Can you work these out from the model? Positions are in its coordinate system, mm. Face numbers are marked on the shaded views. A direction names the side the tool comes from. Round coordinates to 2 decimals unless told otherwise and drop trailing zeros. Order: outer loops, then holes, each group sorted by start corner. A loop starts at its lowest first (then second) coordinate and runs counter-clockwise, first axis right, second up. Notation, with made-up numbers: (-28, -28.75) -> (3, -28.75) arc R24 cw to (3, -16.75) -> close; hole circle Ø5 at (-1, 78). An arc over 180 degrees is marked (long way). Use a Markdown table: item, result. Add a question column.
Q1. For the marked faces 1, 2, 3, 4 and 5, which set-ups out of +Z, -Z, +X, -X, +Y, -Y let a thin tool reach every point of the face, with its end or its side?
Q2. I'm going to push flat-ended pins straight in: pin 1 Ø15 at (x, y) = (13, 13.5) entering from +Z; pin 2 Ø1.8 at (x, y) = (-50, 14) entering from +Z; pin 3 Ø2 at (y, z) = (9.5, -22) entering from +X. Where does each tip first touch, or does it pass through?
Q3. If we section it at C-C on x = -34.5: List the corners of the cut face in (y, z) for me, plus the area to 3 significant figures.
Q4. If we section it at D-D on z = -5: List the corners of the cut face in (x, y) for me.
Q5. We'd pull the mould along X, two halves only. Please class the marked faces 6, 7 and 8: +X half, -X half, draft (parallel to the pull), parting line (faces both ways), or undercut.
Q6. If we section it at A-A on z = 8.5: List the corners of the cut face in (x, y) for me.
Q7. I need wall thicknesses on line 1 along X through (y, z) = (12, 45.5); line 2 along X through (y, z) = (2.5, 21.5); line 3 along Z through (x, y) = (-25, 3). Which ranges of each line are inside material? Lowest first, please. Write a range as [from, to].
Q8. If we section it at B-B on y = 11: List the corners of the cut face in (x, z) for me, plus the area to 3 significant figures.
```python
from build123d import *

# Parameters (mm, degrees)
AUFSATZ_LINEAR_AUSTRAGEN1_DEPTH = 30
SKIZZE5_W                       = 8.1
SKIZZE5_H                       = 30
AUFSATZ_LINEAR_AUSTRAGEN2_DEPTH = 3
FASE2_SIZE                      = 0.5
VERRUNDUNG1_R                   = 5
VERRUNDUNG2_R                   = 10
SCHNITT_LINEAR_AUSTRAGEN1_DEPTH = 135.433068848
VERRUNDUNG3_R                   = 2
SCHNITT_LINEAR_AUSTRAGEN2_DEPTH = 97.953597148
SCHNITT_LINEAR_AUSTRAGEN3_DEPTH = 103.097992145


with BuildPart() as part:
    # Skizze1 → Aufsatz-Linear austragen1 (new body)
    with BuildSketch(Plane(origin=(0, 0, 0), x_dir=(1, 0, 0), z_dir=(0, 1, 0))):
        Polygon((-56.5, 0), (-56.5, -26), (-46.5, -26), (-46.5, 8), (60, 8), (60, -60), (70, -60), (70, 0), (70, 20), (-56.5, 20), align=None)
    extrude(amount=AUFSATZ_LINEAR_AUSTRAGEN1_DEPTH)

    # Skizze5 → Aufsatz-Linear austragen2 (add)
    with BuildSketch(Plane(origin=(0, 0, -20), x_dir=(-1, 0, 0), z_dir=(0, 0, -1))):
        with Locations((0, 15)):
            Rectangle(SKIZZE5_W, SKIZZE5_H)
    extrude(amount=AUFSATZ_LINEAR_AUSTRAGEN2_DEPTH)

    # Fase2
    fase2_edges = [part.edges().sort_by_distance(p)[0] for p in [
        (-4.05, 15, -23),
        (0, 0, -23),
        (4.05, 15, -23),
        (0, 30, -23),
    ]]
    chamfer(fase2_edges, length=FASE2_SIZE)

    # Verrundung1
    verrundung1_edges = [part.edges().sort_by_distance(p)[0] for p in [
        (70, 15, -20),
        (-56.5, 15, -20),
    ]]
    fillet(verrundung1_edges, radius=VERRUNDUNG1_R)

    # Verrundung2
    verrundung2_edges = [part.edges().sort_by_distance(p)[0] for p in [
        (60, 15, -8),
        (-46.5, 15, -8),
    ]]
    fillet(verrundung2_edges, radius=VERRUNDUNG2_R)

    # Skizze8 → Schnitt-Linear austragen1 (cut, through all)
    with BuildSketch(Plane.ZY.offset(-60)):
        Polygon((17, 26.65), (15.35, 25), (17, 23.35), (18.65, 25), align=None)
        Polygon((48.35, 25), (50, 26.65), (51.65, 25), (50, 23.35), align=None)
    extrude(amount=-SCHNITT_LINEAR_AUSTRAGEN1_DEPTH, mode=Mode.SUBTRACT)

    # Verrundung3
    verrundung3_edges = [part.edges().sort_by_distance(p)[0] for p in [
        (70, 15, 60),
        (60, 15, 60),
        (-46.5, 15, 26),
        (-56.5, 15, 26),
    ]]
    fillet(verrundung3_edges, radius=VERRUNDUNG3_R)

    # Skizze9 → Schnitt-Linear austragen2 (cut, through all)
    with BuildSketch(Plane(origin=(0, 0, 0), x_dir=(0, 0, -1), z_dir=(1, 0, 0))):
        Polygon((-16, 27.192031022), (-13.807968978, 25), (-16, 22.807968978), (-18.192031022, 25), align=None)
        Polygon((-16, 7.192031022), (-13.807968978, 5), (-16, 2.807968978), (-18.192031022, 5), align=None)
    extrude(amount=-SCHNITT_LINEAR_AUSTRAGEN2_DEPTH, mode=Mode.SUBTRACT)

    # Skizze10 → Schnitt-Linear austragen3 (cut, through all)
    with BuildSketch(Plane.XY.offset(-8)):
        Polygon((0, 17.55), (2.55, 15), (0, 12.45), (-2.55, 15), align=None)
    extrude(amount=-SCHNITT_LINEAR_AUSTRAGEN3_DEPTH, mode=Mode.SUBTRACT)


solid = part.part
```
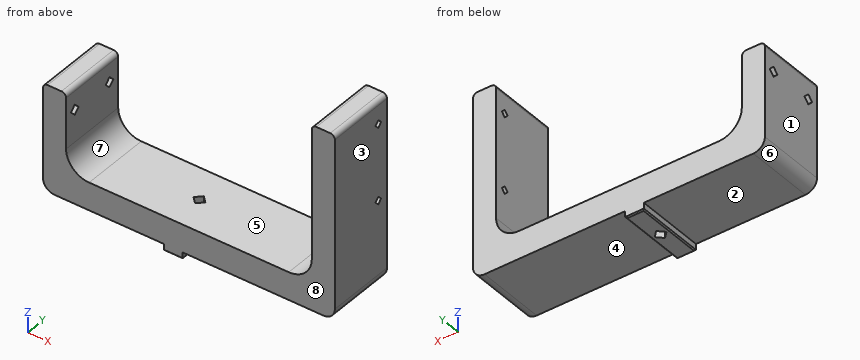
Answer below:
| question | item | result |
|---|---|---|
| 1 | face 1 | +Z, -Z, -X, +Y, -Y |
| 1 | face 2 | -Z, -X, +Y, -Y |
| 1 | face 3 | +Z, -Z, +X, +Y, -Y |
| 1 | face 4 | -Z, +X, +Y, -Y |
| 1 | face 5 | +Z, +Y, -Y |
| 2 | pin 1 | z = -8 |
| 2 | pin 2 | z = 26 |
| 2 | pin 3 | x = 4.05 |
| 3 | outline | (0, -20) -> (30, -20) -> (30, -8) -> (0, -8) -> close |
| 3 | area | 360 mm² |
| 4 | outline | (-56.5, 0) -> (-43.64, 0) -> (-43.64, 30) -> (-56.5, 30) -> close; (57.14, 0) -> (70, 0) -> (70, 30) -> (57.14, 30) -> close |
| 5 | face 6 | -X half |
| 5 | face 7 | undercut |
| 5 | face 8 | draft |
| 6 | outline | (-56.5, 0) -> (-46.5, 0) -> (-46.5, 30) -> (-56.5, 30) -> close; (60, 0) -> (70, 0) -> (70, 30) -> (60, 30) -> close |
| 7 | line 1 | [60, 70] |
| 7 | line 2 | [-56.5, -46.5], [60, 70] |
| 7 | line 3 | [-20, -8] |
| 8 | outline | (-56.5, -15) arc R5 ccw to (-51.5, -20) -> (-4.05, -20) -> (-4.05, -22.5) -> (-3.55, -23) -> (3.55, -23) -> (4.05, -22.5) -> (4.05, -20) -> (65, -20) arc R5 ccw to (70, -15) -> (70, 58) arc R2 ccw to (68, 60) -> (62, 60) arc R2 ccw to (60, 58) -> (60, 2) arc R10 cw to (50, -8) -> (-36.5, -8) arc R10 cw to (-46.5, 2) -> (-46.5, 24) arc R2 ccw to (-48.5, 26) -> (-54.5, 26) arc R2 ccw to (-56.5, 24) -> close |
| 8 | area | 2,590 mm² |
